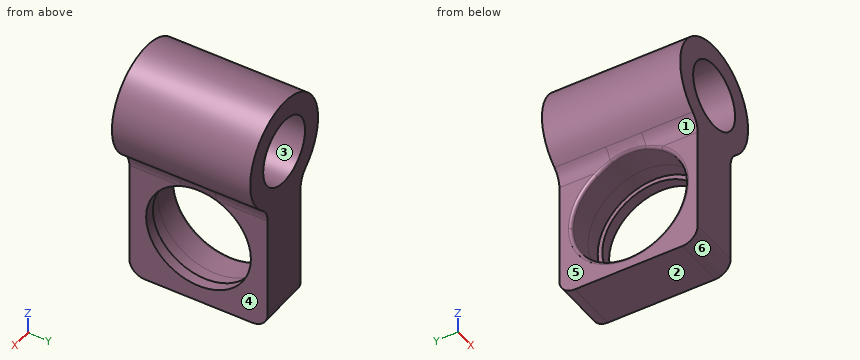
from build123d import *

# Parameters (mm, degrees)
F0_W          = 45
F0_H          = 45
F0_R          = 18.55
F0_R_2        = 17.05
F2_DEPTH      = 8.5
F1_R          = 17.5
F1_R_2        = 10.8
F3_DEPTH      = 22.5
F4_DEPTH      = 22.5
F5_R          = 7
F6_DEPTH      = 25
F6_DEPTH_BACK = 5
F7_R          = 1
F8_R          = 5


with BuildPart() as f2:
    # F0 (on Right) → F2 (new body, symmetric)
    with BuildSketch(Plane.YZ):
        Rectangle(F0_W, F0_H)
        Circle(F0_R, mode=Mode.SUBTRACT)
        Circle(F0_R)
        Circle(F0_R_2, mode=Mode.SUBTRACT)
    extrude(amount=F2_DEPTH, both=True)

    # F1 (on Front) → F3 (join, symmetric)
    with BuildSketch(Plane.XZ):
        with Locations((0, 35)):
            Circle(F1_R)
        with Locations((0, 35)):
            Circle(F1_R_2, mode=Mode.SUBTRACT)
        with Locations((0, 35)):
            Circle(F1_R_2)
    extrude(amount=F3_DEPTH, both=True)

    # F1 (on Front) → F4 (cut, symmetric)
    with BuildSketch(Plane.XZ):
        with Locations((0, 35)):
            Circle(F1_R_2)
    extrude(amount=F4_DEPTH, both=True, mode=Mode.SUBTRACT)

    # F5
    f5_edges = [f2.edges().sort_by_distance(p)[0] for p in [
        (-8.5, 0, 19.702941),
        (8.5, 0, 19.702941),
    ]]
    fillet(f5_edges, radius=F5_R)

    # F0 (on Right) → F6 (cut, two sides)
    with BuildSketch(Plane.YZ) as f6_sk:
        Circle(F0_R)
        Circle(F0_R_2, mode=Mode.SUBTRACT)
    extrude(amount=-F6_DEPTH, mode=Mode.SUBTRACT)
    extrude(f6_sk.sketch, amount=F6_DEPTH_BACK, mode=Mode.SUBTRACT)

    # F7
    f7_edges = [f2.edges().sort_by_distance(p)[0] for p in [
        (-8.5, -9.241811, -16.083887),
        (-8.5, 16.083887, 9.241811),
        (-8.912254, 0, 18.55),
    ]]
    fillet(f7_edges, radius=F7_R)

    # F8
    f8_edges = [f2.edges().sort_by_distance(p)[0] for p in [
        (0, 22.5, -22.5),
        (0, -22.5, -22.5),
    ]]
    fillet(f8_edges, radius=F8_R)


solid = f2.part
Can you work these out from the model? Positions are in its coordinate system, mm. Face numbers are marked on the shaded views. A direction names the side the tool comes from. Round coordinates to 2 decimals unless told otherwise and drop trailing zeros. Loops run counter-clockwise (first coordinate to the right, second up) from the corner with the lowest first, then second, coordinate; pieces in that order, holes last. Notation, with made-up numbers: (-3, 49.25) - (40, 49.25) arc R16 cw to (40, 76.25) - close; hole circle Ø6 at (-36.5, 88.5). An arc over 180 degrees is marked (long way). Use CSV: the item, a comma, the result in double quotes. Start each with the question number.
1) We'd pull the mould along X, two halves only. Please class the marked faces 1, 2 and 3: released by +X, released by -X, zero draft, split by the parting line, or undercut.
2) If we section it at C-C on x = -15: Write out the boundary of the cut face in (y, z).
3) If we section it at A-A on z = 35: Write out the boundary of the cut face in (x, y), plus the area to 3 significant figures.
4) For the marked faces 4, 5 and 6, which set-ups out of +Z, -Z, +X, -X, +Y, -Y let a thin tool reach every point of the face, with its end or its side?
5) Please list where these lines run through material, in increasing order: probe 1 along Y at (x, z) = (-3, 0); probe 2 along X at (y, z) = (-2.5, 35.5); probe 3 along Z at (x, y) = (-4.75, 0). Write a range as [from, to].
6) If we section it at B-B on y = 0: Count the separate pieces of the cut face and the enclosed holes in it, plus the area to 3 significant figures.
7) For pin 1 Ø10 at (y, z) = (-15.5, -11) entering from +X; pin 2 Ø4 at (y, z) = (3, 15) entering from -X; pin 3 Ø1.5 at (y, z) = (11.5, 9) entering from -X; pin 4 Ø1 at (x, y) = (5, 2.5) entering from +Z, each with a flat end and sliding along its axis, tell me the tip position at first contact or that it passes through.
Geometry results:
1,face 1,"released by -X"
1,face 2,"zero draft"
1,face 3,"undercut"
2,outline,"(-22.5, 25.99) - (22.5, 25.99) - (22.5, 44.01) - (-22.5, 44.01) - close"
3,outline,"(-17.5, -22.5) - (-10.8, -22.5) - (-10.8, 22.5) - (-17.5, 22.5) - close; (10.8, -22.5) - (17.5, -22.5) - (17.5, 22.5) - (10.8, 22.5) - close"
3,area,"603 mm2"
4,face 4,"-Z, +X, +Y, -Y"
4,face 5,"-Z, -X, +Y, -Y"
4,face 6,"-Z, +X, -X, -Y"
5,probe 1,"y = [-22.5, -18.55], [18.55, 22.5]"
5,probe 2,"x = [-17.49, -10.79], [10.79, 17.49]"
5,probe 3,"z = [-22.5, -18.55], [18.55, 25.3], [44.7, 51.84]"
6,separate pieces,"2"
6,enclosed holes,"1"
6,area,"670 mm2"
7,pin 1,"stops at x = 8.5"
7,pin 2,"stops at x = 5"
7,pin 3,"passes through"
7,pin 4,"stops at z = 51.91"
